Geometry check sheet. Reference: the model listing, model coordinates, mm. Round coordinates to 2 decimals unless told otherwise and drop trailing zeros. Write each loop counter-clockwise with the first axis right and the second up, starting at its lowest first coordinate (ties: lowest second). Pieces come first, ordered by that corner, then holes. Notation, with made-up numbers: (10, 31.25) - (48, 31.25) arc R15 cw to (48, 44.25) - close; hole circle Ø6 at (1.25, 68.5). An arc over 180 degrees is marked (long way). Return JSON: item names as keys, results as strings.
```python
from build123d import *

# Parameters (mm, degrees)
SKETCH1_W           = 99.25
SKETCH1_H           = 4.25
BOSS_EXTRUDE1_DEPTH = 25
CUT_EXTRUDE1_START  = 43.476884
SKETCH2_R           = 7.5
CUT_EXTRUDE1_DEPTH  = 6


with BuildPart() as part:
    # Sketch1 → Boss-Extrude1 (new, symmetric)
    with BuildSketch(Plane.XY):
        with Locations((-4.860782361, 41.351884068)):
            Rectangle(SKETCH1_W, SKETCH1_H)
    extrude(amount=BOSS_EXTRUDE1_DEPTH, both=True)

    # Sketch2 → Cut-Extrude1 (cut)
    with BuildSketch(Plane(origin=(0, 0, 0), x_dir=(1, 0, 0), z_dir=(0, 1, 0)).offset(CUT_EXTRUDE1_START)):
        with Locations(Location((-4.869275063, 4.996031553, 0), (0, 0, 270))):
            Circle(SKETCH2_R)
    extrude(amount=-CUT_EXTRUDE1_DEPTH, mode=Mode.SUBTRACT)


solid = part.part
```
(1) Release check for a two-part mould opening along X. For faces 1 (the face through (44.764, 41, 0)), 2 (the face through (-6, 39.227, 6)), 3 (the face through (-54.486, 41, 0)), 4 (the face through (-7.742, 41.382, 1.932)) record: pulls with the +X half, pulls with the -X half, needs draft (parallel to the pull), parting line crosses it, or undercut.
Response values:
{"face 1": "pulls with the +X half", "face 2": "needs draft", "face 3": "pulls with the -X half", "face 4": "undercut"}
(2) Material ranges on line 1 along Z through (x, y) = (-6, 41); line 2 along Z through (x, y) = (-10.5, 39.5); line 3 along X through (y, z) = (39.8, -3.5), recorded low to high. Write a range as [from, to].
Response values:
{"line 1": "z = [-25, -12.41], [2.42, 25]", "line 2": "z = [-25, -9.95], [-0.04, 25]", "line 3": "x = [-54.49, -12.22], [2.48, 44.76]"}
(3) Section check B-B, the plane y = 40.95. Enter the section's corners in (x, z), plus the area to 3 significant figures.
Response values:
{"outline": "(-54.49, -25) - (44.76, -25) - (44.76, 25) - (-54.49, 25) - close; hole circle Ø15 at (-4.87, -5)", "area": "4,790 mm^2"}
(4) Section check A-A, the plane z = -5. Enter the section's corners in (x, y).
Response values:
{"outline": "(-54.49, 39.23) - (-12.37, 39.23) - (-12.37, 43.48) - (-54.49, 43.48) - close; (2.63, 39.23) - (44.76, 39.23) - (44.76, 43.48) - (2.63, 43.48) - close"}
(5) Gauge pin test, flat end, axial feed: pin 1 (13.5 mm diameter, centred on x = -4.87, z = -5, fed in from +Y). Record the tip position at first contact, or that the pin passes through.
Response values:
{"pin 1": "passes through"}
